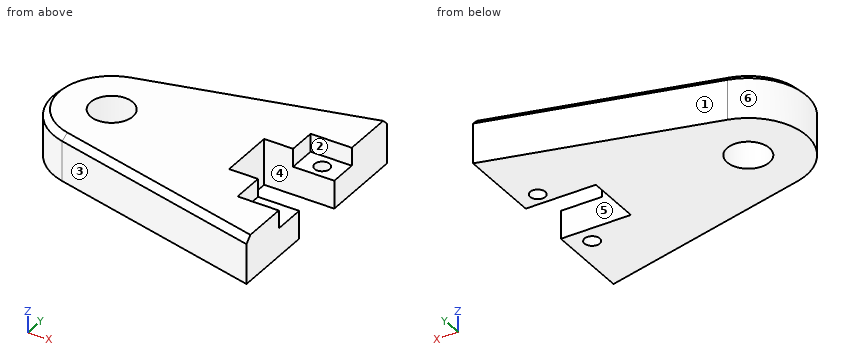
```python
from build123d import *

# Parameters (mm, degrees)
SKETCH_R        = 10.561309
PAD_DEPTH       = 23
SKETCH001_W     = 33.65596
SKETCH001_H     = 57.798376
POCKET_DEPTH    = 9
CHAMFER_SIZE    = 3
SKETCH002_R     = 3.792362
POCKET001_DEPTH = 16


with BuildPart() as part:
    # Sketch → Pad (new body)
    with BuildSketch(Plane.XY):
        with BuildLine():
            Line((101.683037, 56.508842), (-7.323339, 28.107179))
            ThreePointArc((-7.323339, 28.107179), (-29.044704, -0.223526), (-6.889876, -28.216563))
            Line((-6.889876, -28.216563), (101.683037, -54.727728))
            Line((101.683037, -54.727728), (101.683037, -12.993235))
            Line((101.683037, -12.993235), (66.739337, -12.993235))
            Line((66.739337, -12.993235), (66.739337, 14.774349))
            Line((66.739337, 14.774349), (101.683037, 14.774349))
            Line((101.683037, 14.774349), (101.683037, 56.508842))
        make_face()
        Circle(SKETCH_R, mode=Mode.SUBTRACT)
    extrude(amount=PAD_DEPTH)

    # Sketch001 (on Face11 of Pad) → Pocket (cut)
    with BuildSketch(Plane.XY.offset(23)):
        with Locations((97.992905, -0.272637)):
            Rectangle(SKETCH001_W, SKETCH001_H)
    extrude(amount=-POCKET_DEPTH, mode=Mode.SUBTRACT)

    # Chamfer
    chamfer_edges = [part.edges().sort_by_distance(p)[0] for p in [
        (47.39658, -41.472145, 23),
        (-29.044704, -0.223526, 23),
        (47.179849, 42.30801, 23),
    ]]
    chamfer(chamfer_edges, length=CHAMFER_SIZE)

    # Sketch002 (on Face20 of Chamfer) → Pocket001 (cut)
    with BuildSketch(Plane.XY.offset(14)):
        with Locations((91.437004, -21.51132)):
            Circle(SKETCH002_R)
    pocket001 = extrude(amount=-POCKET001_DEPTH, mode=Mode.SUBTRACT)

    # Mirrored: Pocket001 across XZ
    add(pocket001.mirror(Plane.XZ), mode=Mode.SUBTRACT)


solid = part.part
```
Build history of the part. All positions in model axes, mm. Face numbers are marked on the shaded views. A direction names the side the tool comes from. Round coordinates to 2 decimals unless told otherwise and drop trailing zeros. Order: outer loops, then holes, each group sorted by start corner. A loop starts at its lowest first (then second) coordinate and runs counter-clockwise, first axis right, second up. Notation, with made-up numbers: (13.5, -34) - (60.5, -34) arc R22 cw to (60.5, -28) - close; hole circle Ø6 at (80.25, 79.5). An arc over 180 degrees is marked (long way). Use a Markdown table: item, result.
1) Saw through at A-A on z = 15.5. Write the cut outline in (x, y), and give its area (3 significant figures).
Recorded:
| item | result |
|---|---|
| outline | (-7.32, 28.11) arc R29.05 ccw to (-6.89, -28.22) - (101.68, -54.73) - (101.68, -29.17) - (81.16, -29.17) - (81.16, -12.99) - (66.74, -12.99) - (66.74, 14.77) - (81.16, 14.77) - (81.16, 28.63) - (101.68, 28.63) - (101.68, 56.51) - close; hole circle Ø21.12 at (0, 0) |
| area | 8,090 mm² |
2) Pull direction Y, two halves, no side cores. Call the marked faces 1, 2, 3 and 4: pulls with the +Y half, pulls with the -Y half, needs draft (parallel to the pull), parting line crosses it, or undercut.
Recorded:
| item | result |
|---|---|
| face 1 | pulls with the +Y half |
| face 2 | undercut |
| face 3 | pulls with the -Y half |
| face 4 | undercut |
3) Flat gauge pins, fed straight in: pin 1 Ø17 at (x, y) = (0, 0) entering from +Z; pin 2 Ø4 at (x, z) = (44.5, 5) entering from +Y; pin 3 Ø2.5 at (y, z) = (19, 16.5) entering from +X; pin 4 Ø4 at (x, z) = (-0.5, 8) entering from -Y. Where does each tip first touch, or does it go through?
Recorded:
| item | result |
|---|---|
| pin 1 | passes through |
| pin 2 | stops at y = 42.13 |
| pin 3 | stops at x = 81.16 |
| pin 4 | stops at y = -30.27 |
4) Wall check: L1, parallel to Y at x = 93, z = 1.5; L2, parallel to Y at x = 75, z = 12.25; L3, parallel to Y at x = 0, z = 6.5. Give the ranges that are in metal, low to high.
Recorded:
| item | result |
|---|---|
| L1 | y = -52.61 to -24.97, -18.06 to -12.99, 14.77 to 18.06, 24.97 to 54.25 |
| L2 | y = -48.21 to -12.99, 14.77 to 49.56 |
| L3 | y = -29.9 to -10.56, 10.56 to 30.02 |
5) Tool access for the marked faces 5 and 6: list every direction of +Z, -Z, +X, -X, +Y, -Y with a clear straight run to the whole face (end or side of a thin tool).
Recorded:
| item | result |
|---|---|
| face 5 | +Z, -Z, +X |
| face 6 | +Z, -Z, -X |
6) Saw through at B-B on y = 0. Write the cut outline in (x, z), and give its area (3 significant figures).
Recorded:
| item | result |
|---|---|
| outline | (-29.05, 0) - (-10.56, 0) - (-10.56, 23) - (-26.05, 23) - (-29.05, 20) - close; (10.56, 0) - (66.74, 0) - (66.74, 23) - (10.56, 23) - close |
| area | 1,710 mm² |
7) Saw through at D-D on x = 34. Write the cut outline in (y, z).
Recorded:
| item | result |
|---|---|
| outline | (-38.2, 0) - (38.87, 0) - (38.87, 20) - (35.77, 23) - (-35.11, 23) - (-38.2, 20) - close |
8) Saw through at C-C on x = 0. Write the cut outline in (y, z), and give its area (3 significant figures).
Recorded:
| item | result |
|---|---|
| outline | (-29.9, 0) - (-10.56, 0) - (-10.56, 23) - (-26.81, 23) - (-29.9, 20) - close; (10.56, 0) - (30.02, 0) - (30.02, 20) - (26.92, 23) - (10.56, 23) - close |
| area | 883 mm² |
